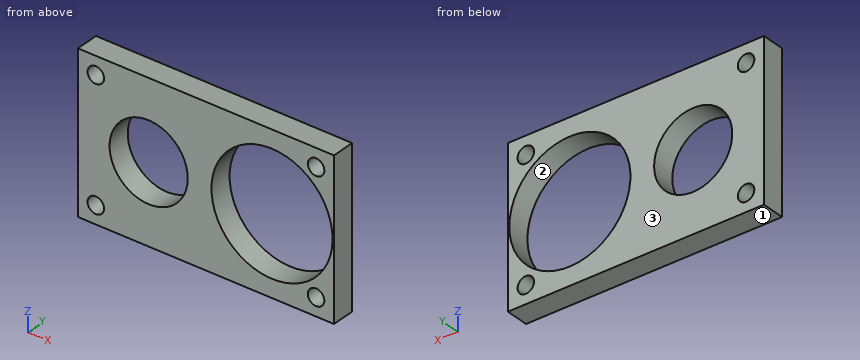
```python
from build123d import *

# Parameters (mm, degrees)
SKETCH11_W          = 46.5
SKETCH11_H          = 28.5
SKETCH11_R          = 1.5
BOSS_EXTRUDE3_DEPTH = 4.2
SKETCH12_R          = 11
CUT_EXTRUDE6_DEPTH  = 5.2
SKETCH13_R          = 7.1
CUT_EXTRUDE7_DEPTH  = 5.2


with BuildPart() as part:
    # Sketch11 → Boss-Extrude3 (new body)
    with BuildSketch(Plane(origin=(0, 0, 0), x_dir=(1, 0, 0), z_dir=(0, 1, 0))):
        with Locations((-5.6, 0)):
            Rectangle(SKETCH11_W, SKETCH11_H)
        with Locations((-25.6, 11)):
            Circle(SKETCH11_R, mode=Mode.SUBTRACT)
        with Locations((14.4, 11)):
            Circle(SKETCH11_R, mode=Mode.SUBTRACT)
        with Locations((14.4, -11)):
            Circle(SKETCH11_R, mode=Mode.SUBTRACT)
        with Locations((-25.6, -11)):
            Circle(SKETCH11_R, mode=Mode.SUBTRACT)
    extrude(amount=-BOSS_EXTRUDE3_DEPTH)

    # Sketch12 → Cut-Extrude6 (cut, through all)
    with BuildSketch(Plane(origin=(0, 0, 0), x_dir=(1, 0, 0), z_dir=(0, 1, 0))):
        with Locations((6.4, 0)):
            Circle(SKETCH12_R)
    extrude(amount=-CUT_EXTRUDE6_DEPTH, mode=Mode.SUBTRACT)

    # Sketch13 → Cut-Extrude7 (cut, through all)
    with BuildSketch(Plane(origin=(0, 0, 0), x_dir=(1, 0, 0), z_dir=(0, 1, 0))):
        with Locations((-16, 0)):
            Circle(SKETCH13_R)
    extrude(amount=-CUT_EXTRUDE7_DEPTH, mode=Mode.SUBTRACT)


solid = part.part
```
Part model, mm, in its own coordinate system. Face numbers are marked on the shaded views. Coordinates: 2 decimals unless noted, no trailing zeros. Order: outer loops, then holes, each group sorted by start corner. A loop starts at its lowest first (then second) coordinate and runs counter-clockwise, first axis right, second up. Notation, with made-up numbers: (21, 19.5) - (75, 19.5) arc R12 ccw to (75, 32.5) - close; hole circle Ø11 at (37.5, 63). An arc over 180 degrees is marked (long way). Return JSON: item names as keys, results as strings. Group by question number.
Item 1: Cut at A-A (x = -25.6). List the corners of the cut face in (y, z), plus the area to 3 significant figures.
Item 2: Cut at D-D (y = -3.2). List the corners of the cut face in (x, z).
Item 3: Pull direction Z, two halves, no side cores. Call the marked faces 1, 2 and 3: pulls with the +Z half, pulls with the -Z half, needs draft (parallel to the pull), parting line crosses it, or undercut.
Item 4: Cut at C-C (z = 0). List the corners of the cut face in (x, y), plus the area to 3 significant figures.
Item 5: Pin check, flat tip, straight feed: pin 1 (1.8 mm diameter, centred on x = -25.6, z = 11, fed in from -Y). Stop position of the tip, or through.
Item 6: Drill centre lines: probe 1 along Z at (x, y) = (14.4, -2.2); probe 2 along Z at (x, y) = (6.4, -2.1); probe 3 along X at (y, z) = (-1.05, -11.75). Where is each one in solid material? Low to high. Write a range as from..to.
Item 7: Cut at B-B (x = -16). List the corners of the cut face in (y, z).
Check values:
{
 "1": {"outline": "(-4.2, -14.25) - (0, -14.25) - (0, -12.5) - (-4.2, -12.5) - close; (-4.2, -9.5) - (0, -9.5) - (0, 9.5) - (-4.2, 9.5) - close; (-4.2, 12.5) - (0, 12.5) - (0, 14.25) - (-4.2, 14.25) - close", "area": "94.5 mm2"},
 "2": {"outline": "(-28.85, -14.25) - (17.65, -14.25) - (17.65, 14.25) - (-28.85, 14.25) - close; hole circle Ø3 at (-25.6, -11); hole circle Ø3 at (-25.6, 11); hole circle Ø14.2 at (-16, 0); hole circle Ø22 at (6.4, 0); hole circle Ø3 at (14.4, -11); hole circle Ø3 at (14.4, 11)"},
 "3": {"face 1": "pulls with the -Z half", "face 2": "undercut", "face 3": "needs draft"},
 "4": {"outline": "(-28.85, -4.2) - (-23.1, -4.2) - (-23.1, 0) - (-28.85, 0) - close; (-8.9, -4.2) - (-4.6, -4.2) - (-4.6, 0) - (-8.9, 0) - close; (17.4, -4.2) - (17.65, -4.2) - (17.65, 0) - (17.4, 0) - close", "area": "43.3 mm2"},
 "5": {"pin 1": "passes through"},
 "6": {"probe 1": "z = -14.25..-12.5, -9.5..-7.55, 7.55..9.5, 12.5..14.25", "probe 2": "z = -14.25..-11, 11..14.25", "probe 3": "x = -28.85..-26.9, -24.3..13.1, 15.7..17.65"},
 "7": {"outline": "(-4.2, -14.25) - (0, -14.25) - (0, -7.1) - (-4.2, -7.1) - close; (-4.2, 7.1) - (0, 7.1) - (0, 14.25) - (-4.2, 14.25) - close"}
}
